from build123d import *

# Parameters (mm, degrees)
SKETCH1_R           = 12
BOSS_EXTRUDE1_DEPTH = 31
SKETCH2_R           = 1.5
CUT_EXTRUDE1_DEPTH  = 5
SKETCH3_R           = 3.25
BOSS_EXTRUDE2_DEPTH = 2
SKETCH4_R           = 1
BOSS_EXTRUDE3_DEPTH = 12
SKETCH5_R           = 2.75
BOSS_EXTRUDE4_DEPTH = 9
CUT_SWEEP6_PITCH    = 1.33


with BuildPart() as part:
    # Sketch1 → Boss-Extrude1 (new body)
    with BuildSketch(Plane(origin=(0, 0, 0), x_dir=(1, 0, 0), z_dir=(0, 1, 0))):
        with Locations(Location((0, 0, 0), (0, 0, 270))):
            Circle(SKETCH1_R)
    extrude(amount=BOSS_EXTRUDE1_DEPTH)

    # Sketch2 → Cut-Extrude1 (cut)
    with BuildSketch(Plane(origin=(0, 31, 0), x_dir=(1, 0, 0), z_dir=(0, 1, 0))):
        with Locations(Location((8, 0, 0), (0, 0, 270))):
            Circle(SKETCH2_R)
        with Locations(Location((-8, 0, 0), (0, 0, 270))):
            Circle(SKETCH2_R)
    extrude(amount=-CUT_EXTRUDE1_DEPTH, mode=Mode.SUBTRACT)

    # Sketch3 → Boss-Extrude2 (add)
    with BuildSketch(Plane(origin=(0, 31, 0), x_dir=(1, 0, 0), z_dir=(0, 1, 0))):
        with Locations(Location((0, 0, 0), (0, 0, 270))):
            Circle(SKETCH3_R)
    extrude(amount=BOSS_EXTRUDE2_DEPTH)

    # Sketch4 → Boss-Extrude3 (add)
    with BuildSketch(Plane(origin=(0, 33, 0), x_dir=(1, 0, 0), z_dir=(0, 1, 0))):
        with Locations(Location((0, 0, 0), (0, 0, 270))):
            Circle(SKETCH4_R)
    extrude(amount=BOSS_EXTRUDE3_DEPTH)

    # Sketch5 → Boss-Extrude4 (add)
    with BuildSketch(Plane(origin=(0, 45, 0), x_dir=(1, 0, 0), z_dir=(0, 1, 0))):
        with Locations(Location((0, 0, 0), (0, 0, 270))):
            Circle(SKETCH5_R)
    extrude(amount=-BOSS_EXTRUDE4_DEPTH)

    # Cut-Sweep6: arcs per turn and ends read off the stored shape
    # Cut-Sweep6: the profile of Sketch6 profile screwed along a left-hand helix through 9 turns, 8 arcs to a turn; built about Z, then put on its axis
    cut_sweep6_z = Axis((0, 0, 0), (0, 0, 1))
    cut_sweep6_corners = [(2.7503, 0, -1.330152512), (1.766472482, 0, -0.83), (2.7503, 0, -0.329847488)]
    with BuildLine(mode=Mode.PRIVATE) as cut_sweep6_profile:
        Line(cut_sweep6_corners[0], cut_sweep6_corners[1])
        Line(cut_sweep6_corners[1], cut_sweep6_corners[2])
        Line(cut_sweep6_corners[2], cut_sweep6_corners[0])
    cut_sweep6_cap = Face(cut_sweep6_profile.wire())
    cut_sweep6_turn_angles = [0, -22.5, -45, -67.5, -90, -112.5, -135, -157.5, -180, -202.5, -225, -247.5, -270, -292.5, -315, -337.5, -360]
    cut_sweep6_turn_weights = [1, 0.9238795325112867, 1, 0.9238795325112867, 1, 0.9238795325112867, 1, 0.9238795325112867, 1, 0.9238795325112867, 1, 0.9238795325112867, 1, 0.9238795325112867, 1, 0.9238795325112867, 1]
    cut_sweep6_turn_rails = [Edge.make_bspline([Vector(p[0], p[1], 0).rotate(cut_sweep6_z, cut_sweep6_turn_angles[k]) / cut_sweep6_turn_weights[k] + Vector(0, 0, p[2] + -CUT_SWEEP6_PITCH * cut_sweep6_turn_angles[k] / 360) for k in range(17)], [0, 0, 0, 1, 1, 2, 2, 3, 3, 4, 4, 5, 5, 6, 6, 7, 7, 8, 8, 8], 2, cut_sweep6_turn_weights) for p in cut_sweep6_corners]
    cut_sweep6_turn_sides = [Face.make_surface_from_curves(cut_sweep6_turn_rails[p[0]], cut_sweep6_turn_rails[p[1]]) for p in [(0, 1), (1, 2), (2, 0)]]
    cut_sweep6 = Plane(origin=(0, 45, 0), x_dir=(-1, 0, 0), z_dir=(0, -1, 0)) * Solid(Shell([*[p.moved(Location((0, 0, CUT_SWEEP6_PITCH * i))) for i in range(9) for p in cut_sweep6_turn_sides], cut_sweep6_cap, cut_sweep6_cap.rotate(cut_sweep6_z, -3240).moved(Location((0, 0, -CUT_SWEEP6_PITCH * -3240 / 360)))]))
    add(cut_sweep6, mode=Mode.SUBTRACT)


solid = part.part
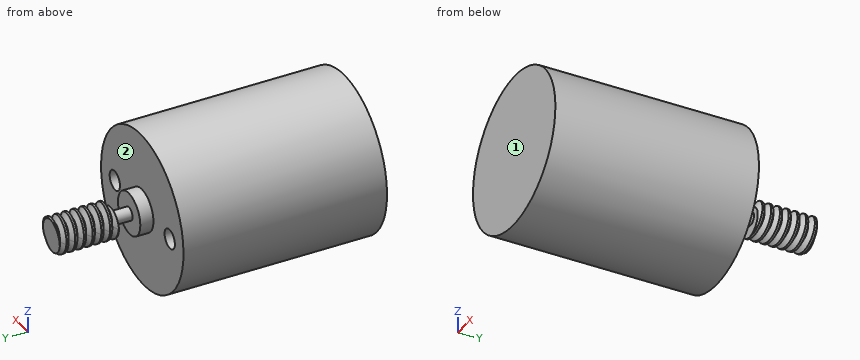
Could you check a few things on this model? Use its own coordinates, in mm. Face numbers are marked on the shaded views. A direction names the side the tool comes from. Give positions to 0.01 mm unless a question says otherwise; leave off trailing zeros. Order: outer loops, then holes, each group sorted by start corner. A loop starts at its lowest first (then second) coordinate and runs counter-clockwise, first axis right, second up. Notation, with made-up numbers: (48, 14.25) -> (54, 14.25) arc R23 cw to (54, 40.25) -> close; hole circle Ø2 at (-37, -33). An arc over 180 degrees is marked (long way). Return JSON: item names as keys, results as strings.
1. I need wall thicknesses on line 1 (X direction, y = 27.35, z = 0); line 2 (Y direction, x = -3.5, z = 3); line 3 (Z direction, x = -0.5, y = 16.5). Which ranges of each line are inside material? Lowest first, please. Write a range as from..to.
Answer list:
{"line 1": "x = -12..-9.5, -6.5..6.5, 9.5..12", "line 2": "y = 0..31", "line 3": "z = -11.99..11.99"}
2. Imagine slicing it at C-C on z = 7. List the corners of the cut face in (x, y) for me.
Answer list:
{"outline": "(-9.75, 0) -> (9.75, 0) -> (9.75, 31) -> (-9.75, 31) -> close"}
3. On a 3-axis mill with a long thin cutter (end or side, diameter ignored), from which of +Z, -Z, +X, -X, +Y, -Y can I reach the whole of each face in a straight line? I mean the marked faces 1 and 2. Say none if no direction works.
Answer list:
{"face 1": "+Z, -Z, +X, -X, -Y", "face 2": "+Y"}
4. Imagine slicing it at B-B on y = 20.5. List the corners of the cut face in (x, z) for me, then the cut area to 3 significant figures.
Answer list:
{"outline": "circle Ø24 at (0, 0)", "area": "452 mm2"}
5. Imagine slicing it at D-D on x = -10.25. List the corners of the cut face in (y, z) for me.
Answer list:
{"outline": "(0, -6.24) -> (31, -6.24) -> (31, 6.24) -> (0, 6.24) -> close"}
6. Imagine slicing it at A-A on x = 8. List the corners of the cut face in (y, z) for me.
Answer list:
{"outline": "(0, -8.94) -> (31, -8.94) -> (31, -1.5) -> (26, -1.5) -> (26, 1.5) -> (31, 1.5) -> (31, 8.94) -> (0, 8.94) -> close"}
7. For pin 1 Ø1 at (x, z) = (-8.5, 3) entering from +Y; pin 2 Ø7 at (x, z) = (3, -5) entering from +Y; pin 3 Ø2.5 at (x, z) = (8, 0) entering from +Y; pin 4 Ø2.5 at (x, z) = (-8, 0) entering from -Y, each with a flat end and sliding along its axis, tell me the tip position at first contact or that it passes through.
Answer list:
{"pin 1": "stops at y = 31", "pin 2": "stops at y = 44.67", "pin 3": "stops at y = 26", "pin 4": "stops at y = 0"}
